from build123d import *

# Parameters (mm, degrees)
SKETCH_1_W          = 20
SKETCH_1_H          = 20
EXTRUDE_1_DEPTH     = 20
SKETCH_2_R          = 6
EXTRUDE_2_DEPTH     = 120
CUT_EXTRUDE_1_DEPTH = 70


with BuildPart() as part:
    # 草图1 → 凸台-拉伸1 (new body)
    with BuildSketch(Plane.XY):
        Rectangle(SKETCH_1_W, SKETCH_1_H)
    extrude(amount=EXTRUDE_1_DEPTH)

    # 草图2 → 凸台-拉伸2 (add)
    with BuildSketch(Plane(origin=(0, 0, 0), x_dir=(-1, 0, 0), z_dir=(0, 0, -1))):
        Circle(SKETCH_2_R)
    extrude(amount=EXTRUDE_2_DEPTH)

    # 草图3 → 切除-拉伸1 (cut)
    with BuildSketch(Plane(origin=(10, 0, 0), x_dir=(0, 0, -1), z_dir=(1, 0, 0))):
        with BuildLine():
            Line((-10, 10), (-23.053143475, 10))
            Line((-23.053143475, 10), (-23.053143475, -10))
            Line((-23.053143475, -10), (-10, -10))
            ThreePointArc((-10, -10), (-20, 0), (-10, 10))
        make_face()
    extrude(amount=-CUT_EXTRUDE_1_DEPTH, mode=Mode.SUBTRACT)


solid = part.part
Geometry check sheet. Reference: the model listing, model coordinates, mm. A direction names the side the tool comes from. Round coordinates to 2 decimals unless told otherwise and drop trailing zeros. Write each loop counter-clockwise with the first axis right and the second up, starting at its lowest first coordinate (ties: lowest second). Pieces come first, ordered by that corner, then holes.
Item 1: Material ranges on line 1 along Z through (x, y) = (-7.25, -0.25); line 2 along Y through (x, z) = (-1.5, -14); line 3 along Z through (x, y) = (7.5, 7), recorded low to high.
Determined:
line 1: z = 0 to 20
line 2: y = -5.81 to 5.81
line 3: z = 0 to 17.14
Item 2: Go/stop test with flat-tipped pins: pin 1 Ø6 at (y, z) = (-4.5, -24) entering from -X; pin 2 Ø8 at (x, z) = (1.5, -49) entering from -Y; pin 3 Ø3 at (x, z) = (6, -5) entering from +Y. Record where each tip stops, or that it passes through.
Determined:
pin 1: stops at x = -5.81
pin 2: stops at y = -6
pin 3: stops at y = 3.97
Item 3: Section check B-B (x = 0). Record the boundary of the cut face in (y, z).
Determined:
outline: (-10, 0) - (-6, 0) - (-6, -120) - (6, -120) - (6, 0) - (10, 0) - (10, 10) arc R10 ccw to (-10, 10) - close
Item 4: Section check C-C (z = -43). Record the boundary of the cut face in (x, y).
Determined:
outline: circle Ø12 at (0, 0)
Item 5: Section check D-D (x = -8). Record the boundary of the cut face in (y, z), plus the area to 3 significant figures.
Determined:
outline: (-10, 0) - (10, 0) - (10, 10) arc R10 ccw to (-10, 10) - close
area: 357 mm2
Item 6: Access from +Z, -Z, +X, -X, +Y, -Y to the whole of each face (thin tool, end or side, straight path). Record for faces 1 (the face through (10, 0, 10)), 2 (the face through (4, 5, 0)).
Determined:
face 1: +Z, -Z, +X, +Y, -Y
face 2: -Z
Item 7: Section check A-A (y = 0). Record the boundary of the cut face in (x, z).
Determined:
outline: (-10, 0) - (-6, 0) - (-6, -120) - (6, -120) - (6, 0) - (10, 0) - (10, 20) - (-10, 20) - close
